from build123d import *

# Parameters (mm, degrees)
SKETCH1_W           = 90
SKETCH1_H           = 40
BOSS_EXTRUDE1_DEPTH = 6
SKETCH2_W           = 28
SKETCH2_H           = 68
CUT_EXTRUDE1_DEPTH  = 4.5
SKETCH6_R           = 1.2
CUT_EXTRUDE5_DEPTH  = 99.671171068
SKETCH7_R           = 1.2
CUT_EXTRUDE6_DEPTH  = 99.671171068
SKETCH8_R           = 2.4
CUT_EXTRUDE7_DEPTH  = 99.591328219
SKETCH9_R           = 2.15
CUT_EXTRUDE8_DEPTH  = 2.4
FILLET3_R           = 1
SKETCH10_W          = 4
SKETCH10_H          = 3
CUT_EXTRUDE9_DEPTH  = 10
FILLET4_R           = 1.5


with BuildPart() as part:
    # Sketch1 → Boss-Extrude1 (new body)
    with BuildSketch(Plane(origin=(0, 0, 0), x_dir=(0, 1, 0), z_dir=(0, 0, 1))):
        with Locations((45, 20)):
            Rectangle(SKETCH1_W, SKETCH1_H)
    extrude(amount=BOSS_EXTRUDE1_DEPTH)

    # Sketch2 → Cut-Extrude1 (cut)
    with BuildSketch(Plane.XY.offset(6)):
        with Locations((-20, 45)):
            Rectangle(SKETCH2_W, SKETCH2_H)
    extrude(amount=-CUT_EXTRUDE1_DEPTH, mode=Mode.SUBTRACT)

    # Sketch6 → Cut-Extrude5 (cut, through all)
    with BuildSketch(Plane.XY.offset(6)):
        with Locations((-20, 85)):
            Circle(SKETCH6_R)
    extrude(amount=-CUT_EXTRUDE5_DEPTH, mode=Mode.SUBTRACT)

    # Sketch7 → Cut-Extrude6 (cut, through all)
    with BuildSketch(Plane.XY.offset(6)):
        with Locations((-20, 5)):
            Circle(SKETCH7_R)
    extrude(amount=-CUT_EXTRUDE6_DEPTH, mode=Mode.SUBTRACT)

    # Sketch8 → Cut-Extrude7 (cut, through all)
    with BuildSketch(Plane.XY.offset(1.5)):
        with Locations((-15.5, 70.7)):
            Circle(SKETCH8_R)
        with Locations((-15.5, 58.7)):
            Circle(SKETCH8_R)
    extrude(amount=-CUT_EXTRUDE7_DEPTH, mode=Mode.SUBTRACT)

    # Sketch9 → Cut-Extrude8 (cut)
    with BuildSketch(Plane(origin=(0, 0, 0), x_dir=(1, 0, 0), z_dir=(0, 0, -1))):
        with Locations(Location((-20, -5, 0), (0, 0, 180))):
            Circle(SKETCH9_R)
        with Locations(Location((-20, -85, 0), (0, 0, 180))):
            Circle(SKETCH9_R)
    extrude(amount=-CUT_EXTRUDE8_DEPTH, mode=Mode.SUBTRACT)

    # Fillet3
    fillet3_edges = [part.edges().sort_by_distance(p)[0] for p in [
        (-40, 45, 0),
        (-20, 90, 0),
        (0, 45, 0),
        (-20, 0, 0),
    ]]
    fillet(fillet3_edges, radius=FILLET3_R)

    # Sketch10 → Cut-Extrude9 (cut)
    with BuildSketch(Plane(origin=(-40, 0, 0), x_dir=(0, -1, 0), z_dir=(-1, 0, 0))):
        with Locations((-45, 4.5)):
            Rectangle(SKETCH10_W, SKETCH10_H)
    extrude(amount=-CUT_EXTRUDE9_DEPTH, mode=Mode.SUBTRACT)

    # Fillet4
    fillet4_edges = [part.edges().sort_by_distance(p)[0] for p in [
        (-37, 47, 3),
        (-37, 43, 3),
    ]]
    fillet(fillet4_edges, radius=FILLET4_R)


solid = part.part
Input: part model. Units: mm. Frame: model coordinates. A direction names the side the tool comes from. Coordinates: 2 decimals unless noted, no trailing zeros. Loops run counter-clockwise (first coordinate to the right, second up) from the corner with the lowest first, then second, coordinate; pieces in that order, holes last.
Q1. Set-up query: faces 3 (the face through (-21.2, 5.05, 4.23)), 4 (the face through (-19.72, 7.13, 1.18)), 5 (the face through (-34, 44.5, 2.8)), 6 (the face through (-37, 47, 5)). Return all of +Z, -Z, +X, -X, +Y, -Y with unobstructed straight access to the full face (end or side cutting, diameter ignored); none if empty.
Q2. Cut plane C-C (x = -7). Output: boundary loops of the cut face in (y, z), then the cut area to 3 significant figures.
Q3. Cut plane A-A (x = -15.5). Output: boundary loops of the cut face in (y, z).
Q4. Contact query for flat-ended pins moving along their axis: pin 1 (8.5 mm diameter, centred on x = -19.5, y = 35.5, fed in from +Z); pin 2 (0.8 mm diameter, centred on x = -37.5, y = 45, fed in from +Z). Output: stop coordinate, or through.
Q5. Cut plane D-D (y = 77). Output: boundary loops of the cut face in (x, z), then the cut area to 3 significant figures.
Q6. Material intervals for line 1 (Y direction, x = -20, z = 1.3); line 2 (Y direction, x = -20, z = 5.25); line 3 (Y direction, x = -15.5, z = 0.85), sorted ascending.
Q7. Cut plane B-B (y = 58.7). Output: boundary loops of the cut face in (x, z), then the cut area to 3 significant figures.
Q8. Draft query along Y for faces 1 (the face through (-20.16, 86.19, 4.23)), 2 (the face through (0, 44, 3)). Return one class per face: +Y half, -Y half, draft (parallel to the pull), parting line (faces both ways), or undercut.
Working result:
1. face 3: +Z, -Z
1. face 4: -Z
1. face 5: +Z
1. face 6: +Z, -X
2. outline: (0, 1) arc R1 ccw to (1, 0) - (89, 0) arc R1 ccw to (90, 1) - (90, 6) - (79, 6) - (79, 1.5) - (11, 1.5) - (11, 6) - (0, 6) - close
2. area: 234 mm2
3. outline: (0, 1) arc R1 ccw to (1, 0) - (56.3, 0) - (56.3, 1.5) - (11, 1.5) - (11, 6) - (0, 6) - close; (61.1, 0) - (68.3, 0) - (68.3, 1.5) - (61.1, 1.5) - close; (73.1, 0) - (89, 0) arc R1 ccw to (90, 1) - (90, 6) - (79, 6) - (79, 1.5) - (73.1, 1.5) - close
4. pin 1: stops at z = 1.5
4. pin 2: stops at z = 3
5. outline: (-40, 1) arc R1 ccw to (-39, 0) - (-1, 0) arc R1 ccw to (0, 1) - (0, 6) - (-6, 6) - (-6, 1.5) - (-34, 1.5) - (-34, 6) - (-40, 6) - close
5. area: 114 mm2
6. line 1: y = 0 to 2.85, 7.15 to 82.85, 87.15 to 90
6. line 2: y = 0 to 3.8, 6.2 to 11, 79 to 83.8, 86.2 to 90
6. line 3: y = 0.01 to 56.3, 61.1 to 68.3, 73.1 to 89.99
7. outline: (-40, 1) arc R1 ccw to (-39, 0) - (-17.9, 0) - (-17.9, 1.5) - (-34, 1.5) - (-34, 6) - (-40, 6) - close; (-13.1, 0) - (-1, 0) arc R1 ccw to (0, 1) - (0, 6) - (-6, 6) - (-6, 1.5) - (-13.1, 1.5) - close
7. area: 106 mm2
8. face 1: undercut
8. face 2: draft
